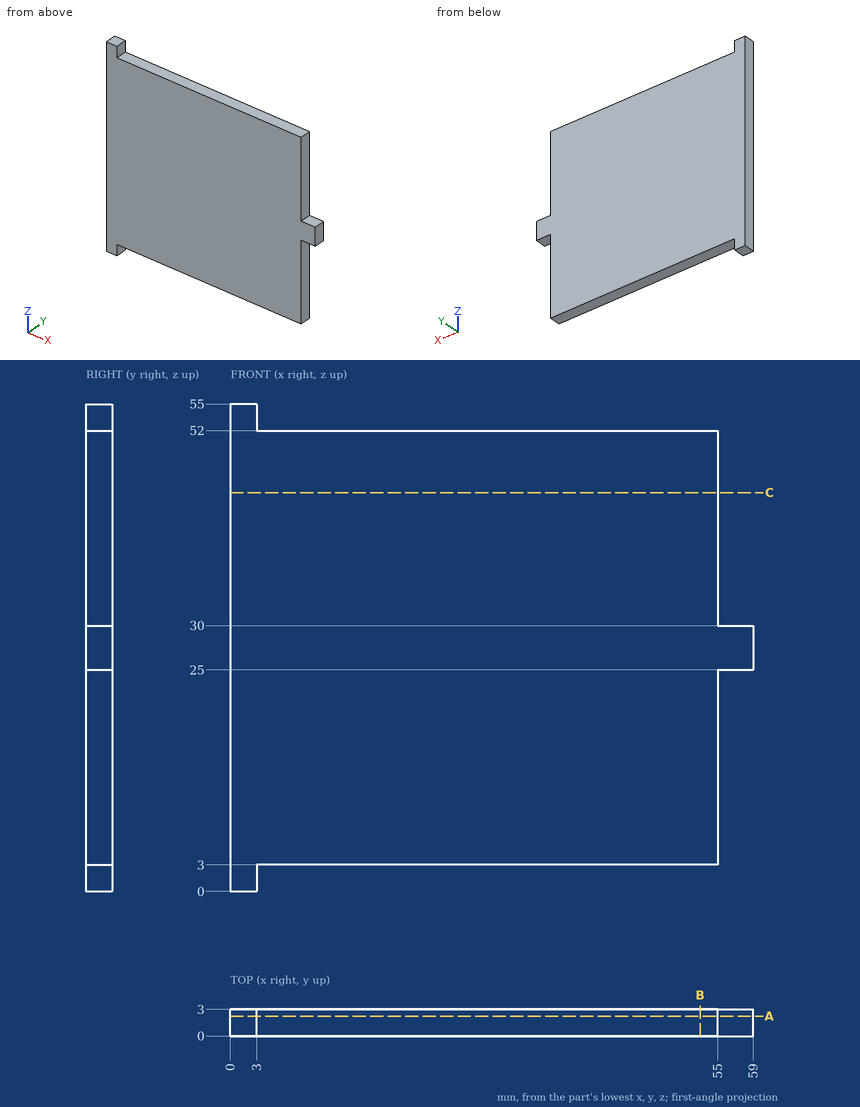
Could you check a few things on this drawing? It's one solid part, dimensions in mm from its lowest x, y, z. Coordinates: 2 decimals unless noted, no trailing zeros. Write each loop counter-clockwise with the first axis right and the second up, starting at its lowest first coordinate (ties: lowest second). Pieces come first, ordered by that corner, then holes. Notation, with made-up numbers: (-29, 17) - (26, 17) arc R23 ccw to (26, 31) - close; hole circle Ø5 at (-2.5, -29). An arc over 180 degrees is marked (long way). Put each result on its own line as item: value. Start each with the question number.
Q1. I want a section at B-B on x = 53. Write out the boundary of the cut face in (y, z), plus the area to 3 significant figures.
Q2. I want a section at A-A on y = 2.25. Write out the boundary of the cut face in (x, z), plus the area to 3 significant figures.
Q3. Please list where these lines run through material, in increasing order: L1, parallel to Z at x = 30, y = 0.5; L2, parallel to X at y = 2.2, z = 24.5.
Q4. I'm going to push flat-ended pins straight in: P1, Ø1.5, axis at y = 0.5, z = 47.5, coming from the -X side; P2, Ø1.5, axis at x = 56, y = 1, coming from the -Z side; P3, Ø1.5, axis at y = 2.5, z = 20.5, coming from the +X side; P4, Ø1.5, axis at x = 57.5, y = 1.5, coming from the +Z side. Where does each tip first touch, or does it pass through?
Q5. I want a section at C-C on z = 45. Write out the boundary of the cut face in (x, y), plus the area to 3 significant figures.
Checks:
1. outline: (0, 3) - (3, 3) - (3, 52) - (0, 52) - close
1. area: 147 mm²
2. outline: (0, 0) - (3, 0) - (3, 3) - (55, 3) - (55, 25) - (59, 25) - (59, 30) - (55, 30) - (55, 52) - (3, 52) - (3, 55) - (0, 55) - close
2. area: 2,730 mm²
3. L1: 3 to 52
3. L2: 0 to 55
4. P1: x = 0
4. P2: z = 25
4. P3: x = 55
4. P4: z = 30
5. outline: (0, 0) - (55, 0) - (55, 3) - (0, 3) - close
5. area: 165 mm²
